Work out the finished part from the listing and answer in its coordinate system (mm). Face numbers are marked on the shaded views. A direction names the side the tool comes from. Round coordinates to 2 decimals unless told otherwise and drop trailing zeros. Loops run counter-clockwise (first coordinate to the right, second up) from the corner with the lowest first, then second, coordinate; pieces in that order, holes last.
```python
from build123d import *

# Parameters (mm, degrees)
CUT_EXTRUDE1_DEPTH = 8
CUT_EXTRUDE2_START = -8
CUT_EXTRUDE2_DEPTH = 8
CIRPATTERN1_COUNT  = 4
CUT_EXTRUDE3_START = -2
CUT_EXTRUDE3_DEPTH = 2


with BuildPart() as part:
    # Sketch1 → Revolve1 (revolve)
    with BuildSketch(Plane(origin=(0, 0, 0), x_dir=(0, 0, -1), z_dir=(1, 0, 0)), mode=Mode.PRIVATE) as revolve1_sk:
        Polygon((0, 15.2), (8.284085908, 15.2), (15.6, 12.517498166), (15.6, 0), (14, 0), (14, 11.4), (8, 13.6), (3, 13.6), (2, 12.8), (1, 12.8), (0, 13.6), align=None)
    revolve(revolve1_sk.sketch.rotate(Axis((0, 0, -14), (0, 0, -1)), 90), axis=Axis((0, 0, -14), (0, 0, -1)))

    # Sketch2 → Cut-Extrude1 (cut)
    with BuildSketch(Plane.XY):
        Polygon((-11.056373105, 15.2), (11.056373105, 15.2), (7.529411765, 10.351229805), (-7.529411765, 10.351229805), align=None)
    extrude(amount=-CUT_EXTRUDE1_DEPTH, mode=Mode.SUBTRACT)

    # Sketch3 → Cut-Extrude2 (cut)
    with BuildSketch(Plane.XY.offset(CUT_EXTRUDE2_START)):
        with BuildLine():
            Line((-8.936632298, 12.295389509), (-7.525585093, 10.354012218))
            Line((-7.525585093, 10.354012218), (-10.354012218, 7.525585093))
            Line((-10.354012218, 7.525585093), (-12.295389509, 8.936632298))
            ThreePointArc((-12.295389509, 8.936632298), (-12.615841165, 8.478239894), (-12.919211808, 8.008368514))
            Line((-12.919211808, 8.008368514), (-11.559294775, 7.165382355))
            ThreePointArc((-11.559294775, 7.165382355), (-13.079877846, 3.725157114), (-13.6, 0))
            Line((-13.6, 0), (0, 0))
            Line((0, 0), (0, 13.6))
            ThreePointArc((0, 13.6), (-3.725483093, 13.079785003), (-7.165958512, 11.558937607))
            Line((-7.165958512, 11.558937607), (-8.009012455, 12.918812619))
            ThreePointArc((-8.009012455, 12.918812619), (-8.478554306, 12.615629865), (-8.936632298, 12.295389509))
        make_face()
    cut_extrude2 = extrude(amount=CUT_EXTRUDE2_DEPTH, mode=Mode.SUBTRACT)

    # CirPattern1: Cut-Extrude2 ×4 about axis
    cirpattern1_axis = Axis((0, 0, 0), (0, 0, 1))
    for i in range(1, CIRPATTERN1_COUNT):
        add(cut_extrude2.rotate(cirpattern1_axis, i * 360 / CIRPATTERN1_COUNT), mode=Mode.SUBTRACT)

    # Sketch4 → Cut-Extrude3 (cut)
    with BuildSketch(Plane.XY.offset(CUT_EXTRUDE3_START)):
        with BuildLine():
            Line((-14.810424985, -3.419256026), (0, 0))
            Line((0, 0), (-14.810424985, 3.419256026))
            ThreePointArc((-14.810424985, 3.419256026), (-15.2, 0), (-14.810424985, -3.419256026))
        make_face()
        with BuildLine():
            Line((14.810424985, 3.419256026), (0, 0))
            Line((0, 0), (14.810424985, -3.419256026))
            ThreePointArc((14.810424985, -3.419256026), (15.2, 0), (14.810424985, 3.419256026))
        make_face()
    extrude(amount=CUT_EXTRUDE3_DEPTH, mode=Mode.SUBTRACT)


solid = part.part
```
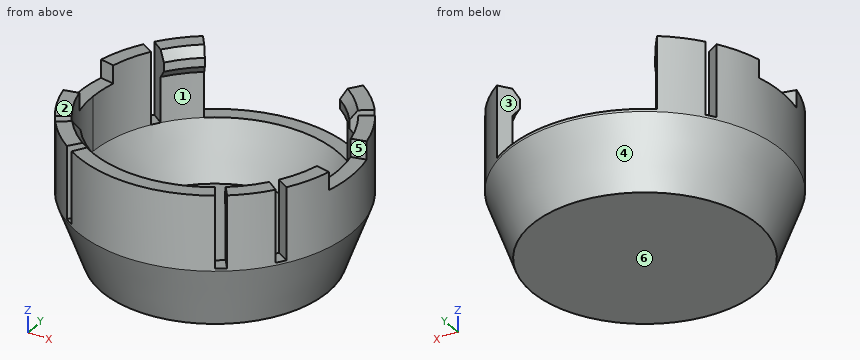
1. Given pin 1 (6 mm diameter, centred on x = 10.5, z = -4.5, fed in from +Y); pin 2 (1.4 mm diameter, centred on x = 8, y = -12, fed in from +Z); pin 3 (2 mm diameter, centred on x = 14.5, y = -0.5, fed in from +Z); pin 4 (4 mm diameter, centred on y = 9, z = -5.5, fed in from -X), each flat-ended and moving along its own axis, determine where each tip first touches the part or whether it passes through.
Answer key:
pin 1: stops at y = 12.29
pin 2: stops at z = 0
pin 3: stops at z = -2
pin 4: stops at x = -13.49
2. Find section A-A (z = -3.75). Write down the section's boundary in (x, y), then the cut area to 3 significant figures.
Answer key:
outline: (-12.92, -8.01) - (-11.56, -7.17) arc R13.6 cw to (-11.56, 7.17) - (-12.92, 8.01) arc R15.2 ccw to start; (-12.3, -8.94) arc R15.2 ccw to (-8.94, -12.3) - (-8, -11) arc R13.6 cw to (-11, -8) - close; (-12.3, 8.94) - (-11, 8) arc R13.6 cw to (-8, 11) - (-8.94, 12.29) arc R15.2 ccw to start; (-8.01, -12.92) arc R15.2 ccw to (8.01, -12.92) - (7.17, -11.56) arc R13.6 cw to (-7.17, -11.56) - close; (8, -11) - (8.94, -12.3) arc R15.2 ccw to (12.3, -8.94) - (11, -8) arc R13.6 cw to start; (8, 11) arc R13.6 cw to (11, 8) - (12.3, 8.94) arc R15.2 ccw to (8.94, 12.29) - close; (11.56, -7.17) - (12.92, -8.01) arc R15.2 ccw to (12.92, 8.01) - (11.56, 7.17) arc R13.6 cw to start
area: 106 mm2
3. Find section C-C (z = -9.75). Write down the section's boundary in (x, y) (1 decimal).
Answer key:
outline: circle Ø29.3 at (0, 0); hole circle Ø25.9 at (0, 0)
4. Consider probe 1 along Z at (x, y) = (6.5, 4); probe 2 along X at (y, z) = (-7, -11.25); probe 3 along Y at (x, z) = (-7, -11). Determine where each line is inside the solid, lowest interval first.
Answer key:
probe 1: z = -15.6 to -14
probe 2: x = -12.25 to -10.25, 10.25 to 12.25
probe 3: y = -12.36 to -10.36, 10.36 to 12.36
5. Find section B-B (x = 0). Write down the section's boundary in (y, z), then the cut area to 3 significant figures.
Answer key:
outline: (-15.2, -8.28) - (-12.52, -15.6) - (12.52, -15.6) - (15.2, -8.28) - (15.2, -8) - (13.6, -8) - (11.4, -14) - (-11.4, -14) - (-13.6, -8) - (-13.6, 0) - (-15.2, 0) - close
area: 74.2 mm2
6. Determine the mould class of the marked faces 1, 2, 3 and 4 for opening direction Y: +Y half, -Y half, draft (parallel to the pull), parting line (faces both ways), or undercut.
Answer key:
face 1: undercut
face 2: draft
face 3: +Y half
face 4: parting line
7. Find section D-D (z = -11.75). Write down the section's boundary in (x, y) (3 decimals), then the cut area to 3 significant figures.
Answer key:
outline: circle Ø27.858 at (0, 0); hole circle Ø24.45 at (0, 0)
area: 140 mm2
8. Which of the six approach directions +Z, -Z, +X, -X, +Y, -Y give full straight-line access (tool end or side, diameter ignored) to the marked faces 5 and 6?
Answer key:
face 5: +Z, +X
face 6: -Z, +X, -X, +Y, -Y
